Design review of the part shown in the three views and the two pictorial views. Dimensions are in mm from the part's minimum x, y and z. A direction names the side the tool comes from. Give positions to 0.01 mm unless a question says otherwise; leave off trailing zeros. Loops run counter-clockwise (first coordinate to the right, second up) from the corner with the lowest first, then second, coordinate; pieces in that order, holes last.
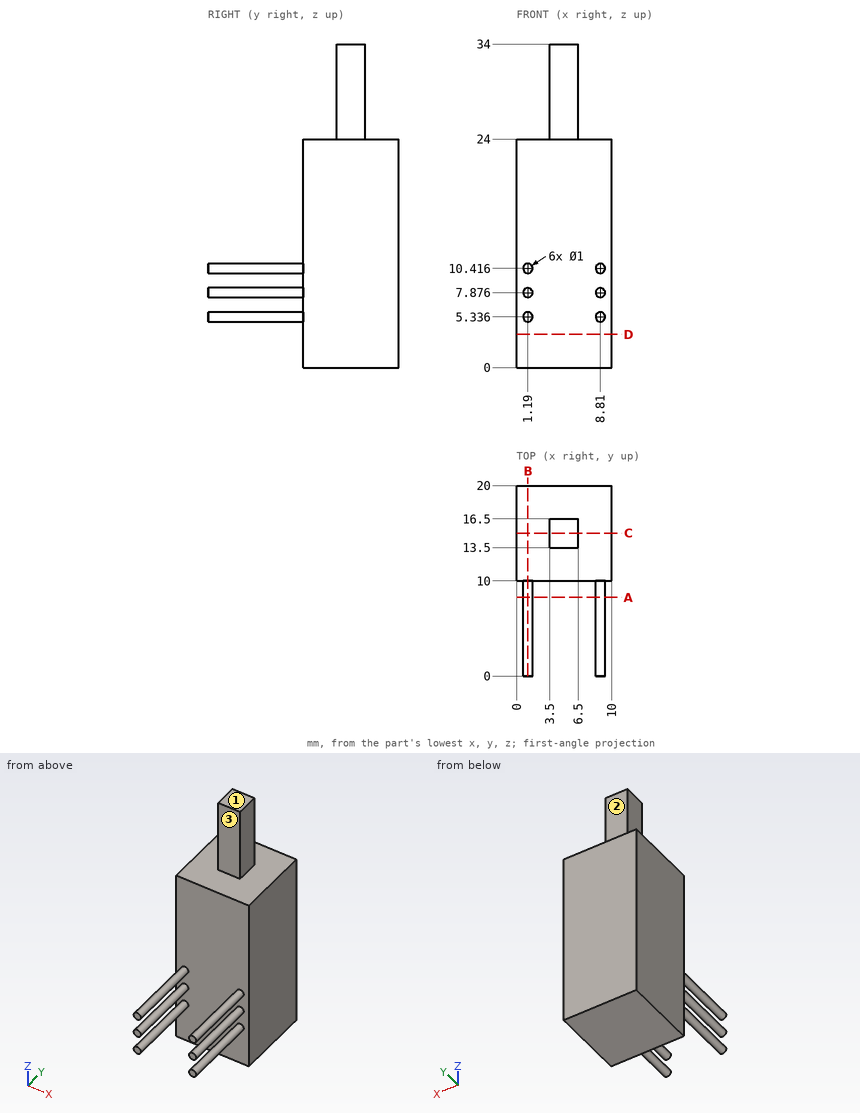
Q1. Consider section B-B on x = 1.19. Give the boundary of the cut face in (y, z) (1 decimal).
Answers:
outline: (0, 4.8) - (10, 4.8) - (10, 0) - (20, 0) - (20, 24) - (10, 24) - (10, 10.9) - (0, 10.9) - (0, 9.9) - (10, 9.9) - (10, 8.4) - (0, 8.4) - (0, 7.4) - (10, 7.4) - (10, 5.8) - (0, 5.8) - close
Q2. Consider section C-C on y = 15. Give the boundary of the cut face in (x, z), plus the area to 3 significant figures.
Answers:
outline: (0, 0) - (10, 0) - (10, 24) - (6.5, 24) - (6.5, 34) - (3.5, 34) - (3.5, 24) - (0, 24) - close
area: 270 mm2
Q3. Consider section D-D on z = 3.5. Give the boundary of the cut face in (x, y), plus the area to 3 significant figures.
Answers:
outline: (0, 10) - (10, 10) - (10, 20) - (0, 20) - close
area: 100 mm2
Q4. For probe 1 along Z at (x, y) = (8.75, 6.75); probe 2 along Y at (x, z) = (1, 4); probe 3 along Z at (x, y) = (8.75, 13), list the stretches that pass through material, from the lowest coordinate up.
Answers:
probe 1: z = 4.84 to 5.83, 7.38 to 8.37, 9.92 to 10.91
probe 2: y = 10 to 20
probe 3: z = 0 to 24
Q5. For pin 1 Ø0.9 at (y, z) = (15, 27.5) entering from +X; pin 2 Ø1 at (y, z) = (5.5, 5.5) entering from +X; pin 3 Ø4 at (x, z) = (9, 12) entering from -Y; pin 4 Ø3 at (x, z) = (6, 10) entering from -Y, all flat-tipped, find the tip position at first contact; note any pin that passes through.
Answers:
pin 1: stops at x = 6.5
pin 2: stops at x = 9.31
pin 3: stops at y = 0
pin 4: stops at y = 10
Q6. Machinability: for the marked faces 1, 2 and 3, which of the approach directions +Z, -Z, +X, -X, +Y, -Y give a long, thin tool a straight path to every point of the face, cutting with its end or side? Answer none if there is none.
Answers:
face 1: +Z, +X, -X, +Y, -Y
face 2: +Z, +X, -X, +Y
face 3: +Z, +X, -X, -Y
Q7. Consider section A-A on y = 8.25. Give the boundary of the cut face in (x, z) (1 decimal).
Answers:
outline: circle Ø1 at (1.2, 5.3); circle Ø1 at (1.2, 7.9); circle Ø1 at (1.2, 10.4); circle Ø1 at (8.8, 5.3); circle Ø1 at (8.8, 7.9); circle Ø1 at (8.8, 10.4)
